```python
from build123d import *

# Parameters (mm, degrees)
BOSS_EXTRUDE1_DEPTH      = 17.9
BOSS_EXTRUDE1_DEPTH_BACK = 17.9
CUT_EXTRUDE1_DEPTH       = 48.206037749
CUT_EXTRUDE1_DEPTH_BACK  = 48.206037749
SKETCH3_W                = 36
SKETCH3_H                = 22
CUT_EXTRUDE2_DEPTH       = 12.5
CUT_EXTRUDE2_DEPTH_BACK  = 12.5
SKETCH4_R                = 7.65
CUT_EXTRUDE3_DEPTH       = 16
CUT_EXTRUDE3_DEPTH_BACK  = 16
SKETCH5_R                = 6.65
CUT_EXTRUDE4_DEPTH       = 16.8
CUT_EXTRUDE4_DEPTH_BACK  = 16.8
SKETCH6_R                = 4.75
CUT_EXTRUDE5_DEPTH       = 48.206037749
CUT_EXTRUDE5_DEPTH_BACK  = 48.206037749
SKETCH7_R                = 3.5
CUT_EXTRUDE6_DEPTH       = 48.206037749
CUT_EXTRUDE6_DEPTH_BACK  = 20.4
CUT_EXTRUDE7_DEPTH       = 48.206037749
CUT_EXTRUDE7_DEPTH_BACK  = 48.206037749
SKETCH11_R               = 2.7
CUT_EXTRUDE8_DEPTH       = 3
SKETCH14_R               = 1.65
CUT_EXTRUDE10_DEPTH      = 33.3
SKETCH15_R               = 2.7
CUT_EXTRUDE11_DEPTH      = 3.3
SKETCH16_W               = 5.75
SKETCH16_H               = 2.05
CUT_EXTRUDE12_DEPTH      = 7.665


with BuildPart() as part:
    # Sketch2 → Boss-Extrude1 (new, two sides: drawn at the far end of the back side and taken through both)
    with BuildSketch(Plane.XY.offset(-BOSS_EXTRUDE1_DEPTH_BACK)):
        with BuildLine():
            Line((-30, -12), (0, -12))
            Line((0, -12), (0, 12))
            Line((0, 12), (-30, 12))
            ThreePointArc((-30, 12), (-42, 0), (-30, -12))
        make_face()
    extrude(amount=BOSS_EXTRUDE1_DEPTH + BOSS_EXTRUDE1_DEPTH_BACK)

    # Sketch3 → Cut-Extrude1 (cut, two sides: drawn at the far end of the back side and taken through both)
    with BuildSketch(Plane(origin=(0, 0, 0), x_dir=(1, 0, 0), z_dir=(0, 1, 0)).offset(-CUT_EXTRUDE1_DEPTH_BACK)):
        with Locations((-24, 0)):
            Rectangle(SKETCH3_W, SKETCH3_H)
    extrude(amount=CUT_EXTRUDE1_DEPTH + CUT_EXTRUDE1_DEPTH_BACK, mode=Mode.SUBTRACT)

    # Sketch4 → Cut-Extrude2 (cut, two sides: drawn at the far end of the back side and taken through both)
    with BuildSketch(Plane.XY.offset(-CUT_EXTRUDE2_DEPTH_BACK)):
        with Locations(Location((-30, 0, 0), (0, 0, 180))):
            Circle(SKETCH4_R)
    extrude(amount=CUT_EXTRUDE2_DEPTH + CUT_EXTRUDE2_DEPTH_BACK, mode=Mode.SUBTRACT)

    # Sketch5 → Cut-Extrude3 (cut, two sides: drawn at the far end of the back side and taken through both)
    with BuildSketch(Plane.XY.offset(-CUT_EXTRUDE3_DEPTH_BACK)):
        with Locations((-30, 0)):
            Circle(SKETCH5_R)
    extrude(amount=CUT_EXTRUDE3_DEPTH + CUT_EXTRUDE3_DEPTH_BACK, mode=Mode.SUBTRACT)

    # Sketch6 → Cut-Extrude4 (cut, two sides: drawn at the far end of the back side and taken through both)
    with BuildSketch(Plane.XY.offset(-CUT_EXTRUDE4_DEPTH_BACK)):
        with Locations((-30, 0)):
            Circle(SKETCH6_R)
    extrude(amount=CUT_EXTRUDE4_DEPTH + CUT_EXTRUDE4_DEPTH_BACK, mode=Mode.SUBTRACT)

    # Sketch7 → Cut-Extrude5 (cut, two sides: drawn at the far end of the back side and taken through both)
    with BuildSketch(Plane.XY.offset(-CUT_EXTRUDE5_DEPTH_BACK)):
        with Locations((-30, 0)):
            Circle(SKETCH7_R)
    extrude(amount=CUT_EXTRUDE5_DEPTH + CUT_EXTRUDE5_DEPTH_BACK, mode=Mode.SUBTRACT)

    # Sketch10 → Cut-Extrude6 (cut, two sides: drawn at the far end of the back side and taken through both)
    with BuildSketch(Plane(origin=(0, 0, 0), x_dir=(0, 0, -1), z_dir=(1, 0, 0)).offset(-CUT_EXTRUDE6_DEPTH_BACK)):
        with BuildLine():
            Line((-17.9, 1.127220032), (-17.9, -1.127220032))
            ThreePointArc((-17.9, -1.127220032), (-15.225, 0), (-17.9, 1.127220032))
        make_face()
        with BuildLine():
            Line((17.9, 1.127220032), (17.9, -1.127220032))
            ThreePointArc((17.9, -1.127220032), (15.225, 0), (17.9, 1.127220032))
        make_face()
    extrude(amount=CUT_EXTRUDE6_DEPTH + CUT_EXTRUDE6_DEPTH_BACK, mode=Mode.SUBTRACT)

    # Sketch11 → Cut-Extrude7 (cut, two sides: drawn at the far end of the back side and taken through both)
    with BuildSketch(Plane(origin=(0, 0, 0), x_dir=(0, 0, -1), z_dir=(1, 0, 0)).offset(-CUT_EXTRUDE7_DEPTH_BACK)):
        with Locations(Location((0, 0, 0), (0, 0, 90))):
            Circle(SKETCH11_R)
    extrude(amount=CUT_EXTRUDE7_DEPTH + CUT_EXTRUDE7_DEPTH_BACK, mode=Mode.SUBTRACT)

    # Sketch12 → Cut-Extrude8 (cut)
    with BuildSketch(Plane.ZY.offset(6)):
        Polygon((-4.705404694, 0), (-2.352702347, -4.075), (2.352702347, -4.075), (4.705404694, 0), (2.352702347, 4.075), (-2.352702347, 4.075), align=None)
    extrude(amount=-CUT_EXTRUDE8_DEPTH, mode=Mode.SUBTRACT)

    # Sketch14 → Cut-Extrude10 (cut)
    with BuildSketch(Plane(origin=(0, 0, -17.9), x_dir=(-1, 0, 0), z_dir=(0, 0, -1))):
        with Locations((18, -7)):
            Circle(SKETCH14_R)
    cut_extrude10 = extrude(amount=-CUT_EXTRUDE10_DEPTH, mode=Mode.SUBTRACT)

    # Sketch15 → Cut-Extrude11 (cut)
    with BuildSketch(Plane(origin=(0, 0, -17.9), x_dir=(-1, 0, 0), z_dir=(0, 0, -1))):
        with Locations((18, -7)):
            Circle(SKETCH15_R)
    cut_extrude11 = extrude(amount=-CUT_EXTRUDE11_DEPTH, mode=Mode.SUBTRACT)

    # Sketch16 → Cut-Extrude12 (cut)
    with BuildSketch(Plane.XZ.offset(12)):
        with Locations((-18, 14.45)):
            Rectangle(SKETCH16_W, SKETCH16_H)
    cut_extrude12 = extrude(amount=-CUT_EXTRUDE12_DEPTH, mode=Mode.SUBTRACT)

    # Mirror1: Cut-Extrude10, Cut-Extrude11, Cut-Extrude12 across plane
    add(cut_extrude10.mirror(Plane.ZX), mode=Mode.SUBTRACT)
    add(cut_extrude11.mirror(Plane.ZX), mode=Mode.SUBTRACT)
    add(cut_extrude12.mirror(Plane.ZX), mode=Mode.SUBTRACT)


solid = part.part
```
Check sheet for the modelled part. Datum: model origin and axes. Units: mm. A direction names the side the tool comes from. Round coordinates to 2 decimals unless told otherwise and drop trailing zeros. Loops run counter-clockwise (first coordinate to the right, second up) from the corner with the lowest first, then second, coordinate; pieces in that order, holes last. Notation, with made-up numbers: (-8.75, 11.5) - (4.25, 11.5) arc R5 ccw to (4.25, 16.5) - close; hole circle Ø2 at (22, 63.5). An arc over 180 degrees is marked (long way). Write item = value, one per line. Start each with the question number.
Q1. Depth check by flat-ended pin: P1, Ø0.6, axis at y = 6.5, z = 14.5, coming from the -X side; P2, Ø3, axis at x = -18, y = -7, coming from the -Z side (3 decimals); P3, Ø6.5, axis at y = -2.5, z = 3, coming from the -X side. Enter the tip coordinate at first touch or a pass-through.
Q2. Release check for a two-part mould opening along Z. For faces 1 (the face through (-20, -7, -14.6)), 2 (the face through (-18, -9, 13.425)), 3 (the face through (-20.494, -8.034, -16.273)) record: pulls with the +Z half, pulls with the -Z half, needs draft (parallel to the pull), parting line crosses it, or undercut.
Q3. Thickness scan on L1, parallel to Y at x = -18, z = 12; L2, parallel to Y at x = -30, z = 16.65; L3, parallel to Z at x = -30, y = 4. Record the ranges inside material, lowest first.
Q4. Section check D-D (x = -18). Count the separate pieces of the cut face and the enclosed holes in it, plus the area to 3 significant figures.
Q5. Section check A-A (z = 0). Record the boundary of the cut face in (x, y) (3 decimals), plus the area to 3 significant figures.
Q6. Access from +Z, -Z, +X, -X, +Y, -Y to the whole of each face (thin tool, end or side, straight path). Record for faces 4 (the face through (-20, 0, -11)), 5 (the face through (-10.343, -0.052, -15.226)), 6 (the face through (-18, 4.335, 14)), 7 (the face through (-5, -4.075, 0)), 8 (the face through (-23.929, 4.655, 11.74)).
Q7. Section check B-B (x = -36). Record the boundary of the cut face in (y, z), plus the area to 3 significant figures.
Q8. Section check C-C (z = -7). Record the boundary of the cut face in (x, y), plus the area to 3 significant figures.
Derived:
q1.P1 = -40.27
q1.P2 = 15.475
q1.P3 = -6
q2.face_1 = pulls with the -Z half
q2.face_2 = undercut
q2.face_3 = needs draft
q3.L1 = -12 to -8.65, -5.35 to 5.35, 8.65 to 12
q3.L2 = -12 to -4.75, 4.75 to 12
q3.L3 = -17.9 to -16.8, 16.8 to 17.9
q4.separate_pieces = 6
q4.enclosed_holes = 0
q4.area = 210 mm^2
q5.outline = (-6, -12) - (0, -12) - (0, -2.7) - (-3, -2.7) - (-3, -4.075) - (-6, -4.075) - close; (-6, 4.075) - (-3, 4.075) - (-3, 2.7) - (0, 2.7) - (0, 12) - (-6, 12) - close
q5.area = 103 mm^2
q6.face_4 = -X, +Y, -Y
q6.face_5 = +X
q6.face_6 = +Y
q6.face_7 = -X
q6.face_8 = none
q7.outline = (-10.39, -17.9) - (10.39, -17.9) - (10.39, -11) - (4.75, -11) - (4.75, -12.5) - (2.87, -12.5) - (2.87, -16) - (-2.87, -16) - (-2.87, -12.5) - (-4.75, -12.5) - (-4.75, -11) - (-10.39, -11) - close; (-10.39, 11) - (-4.75, 11) - (-4.75, 12.5) - (-2.87, 12.5) - (-2.87, 16) - (2.87, 16) - (2.87, 12.5) - (4.75, 12.5) - (4.75, 11) - (10.39, 11) - (10.39, 17.9) - (-10.39, 17.9) - close
q7.area = 218 mm^2
q8.outline = (-6, -12) - (0, -12) - (0, 12) - (-6, 12) - close
q8.area = 144 mm^2
